Verification items for the finished model (mm, model axes). A direction names the side the tool comes from. Give positions to 0.01 mm unless a question says otherwise; leave off trailing zeros. Order: outer loops, then holes, each group sorted by start corner. A loop starts at its lowest first (then second) coordinate and runs counter-clockwise, first axis right, second up. Notation, with made-up numbers: (-9.75, -2.75) - (1.25, -2.75) arc R15 ccw to (1.25, 12.25) - close; hole circle Ø5 at (83.25, 37.25). An arc over 180 degrees is marked (long way). Answer as a JSON object with one key per item and string values. Group by question number.
(1) Section check C-C (x = 1.05). Count the separate pieces of the cut face and the enclosed holes in it, then the cut area to 3 significant figures.
(2) Access from +Z, -Z, +X, -X, +Y, -Y to the whole of each face (thin tool, end or side, straight path). Record for faces 4 (the face through (1.01, 17.4, -18.43)), 5 (the face through (1.01, 29.42, 14.59)), 6 (the face through (0.99, 45.43, 20.85)).
(3) Mould release check, pull along Z, two halves, no side actions. Record for faces 1 (the face through (1, 26, 2)), 2 (the face through (1, 15, -19)), 3 (the face through (0, 33, 0)): +Z half, -Z half, draft (parallel to the pull), parting line (faces both ways), or undercut.
(4) Depth check by flat-ended pin: pin 1 Ø1 at (x, z) = (0.5, -33) entering from +Y; pin 2 Ø0.6 at (x, y) = (1.5, 43) entering from +Z; pin 3 Ø1 at (x, z) = (1, -25.5) entering from -Y. Enter the tip coordinate at first touch or a pass-through.
(5) Thickness scan on line 1 (Z direction, x = 0.15, y = 23.5); line 2 (Z direction, x = 1.2, y = 19.5); line 3 (Y direction, x = 0.85, z = -15). Record the ranges inside material, lowest first.
(6) Section check B-B (y = 51). Record the boundary of the cut face in (x, z), then the cut area to 3 significant figures.
(7) Section check D-D (z = -3.1). Record the boundary of the cut face in (x, y), then the cut area to 3 significant figures.
(8) Section check A-A (y = 21.5). Record the boundary of the cut face in (x, z), then the cut area to 3 significant figures.
```python
from build123d import *

# Parameters (mm, degrees)
EXTRUDE_1_DEPTH        = 2
HOLE_WIZARD_M3_1_D     = 3.2
HOLE_WIZARD_M3_2_D     = 3.2
CHAMFER_1_SIZE         = 15
FILLET_1_R             = 2
CHAMFER_2_SIZE         = 10
SKETCH_6_W             = 8
SKETCH_6_H             = 39
CUT_EXTRUDE_1_DEPTH    = 100
FILLET_2_R             = 1
FILLET_3_R             = 2
FILLET_2_OF_MIRROR_2_R = 1
FILLET_3_OF_MIRROR_2_R = 2
SKETCH_8_R             = 1
CUT_EXTRUDE_2_DEPTH    = 10
FILLET_4_R             = 1
FILLET_5_R             = 10
FILLET_6_R             = 1


with BuildPart() as part:
    # 草图1 → 凸台-拉伸1 (new body)
    with BuildSketch(Plane(origin=(0, 0, 0), x_dir=(0, 0, -1), z_dir=(1, 0, 0))):
        Polygon((0, 50), (26, 50), (26, 54), (32, 54), (32, 50), (35, 50), (35, 30), (14, 30), (14, 18), (19, 18), (19, 0), (0, 0), align=None)
    extrude_1 = extrude(amount=EXTRUDE_1_DEPTH)

    # 镜向1: 凸台-拉伸1 across plane
    add(extrude_1.mirror(Plane(origin=(2, 0, 0), x_dir=(1, 0, 0), z_dir=(0, 0, -1))))

    # M3 间隙孔1 (through all)
    with Locations(Plane(origin=(2, 0, 0), x_dir=(0, 0, -1), z_dir=(1, 0, 0))):
        with Locations((-15.25, 44), (-15.25, 13.5), (15.25, 13.5), (15.25, 44)):
            Hole(HOLE_WIZARD_M3_1_D / 2)

    # M3 间隙孔2 (through all)
    with Locations(Plane(origin=(2, 0, 0), x_dir=(0, 0, -1), z_dir=(1, 0, 0))):
        with Locations((-3.1, 3), (3.1, 3)):
            Hole(HOLE_WIZARD_M3_2_D / 2)

    # 倒角1
    chamfer_1_edges = [part.edges().sort_by_distance(p)[0] for p in [
        (1, 30, -35),
        (1, 30, 35),
    ]]
    chamfer(chamfer_1_edges, length=CHAMFER_1_SIZE)

    # 圆角1
    fillet_1_edges = [part.edges().sort_by_distance(p)[0] for p in [
        (1, 30, -14),
        (1, 18, -14),
        (1, 18, -19),
        (1, 30, 14),
        (1, 18, 14),
        (1, 18, 19),
    ]]
    fillet(fillet_1_edges, radius=FILLET_1_R)

    # 倒角2
    chamfer_2_edges = [part.edges().sort_by_distance(p)[0] for p in [
        (1, 0, -19),
        (1, 0, 19),
    ]]
    chamfer(chamfer_2_edges, length=CHAMFER_2_SIZE)

    # 草图6 → 切除-拉伸1 (cut)
    with BuildSketch(Plane(origin=(2, 0, 0), x_dir=(0, 0, -1), z_dir=(1, 0, 0))):
        with Locations((-6, 26.5)):
            Rectangle(SKETCH_6_W, SKETCH_6_H)
        Polygon((-30.343145751, 46), (-18.343145751, 34), (-12.343145751, 34), (-20.25, 41.906854249), (-20.25, 46), (-24.343145751, 46), align=None)
    cut_extrude_1 = extrude(amount=-CUT_EXTRUDE_1_DEPTH, mode=Mode.SUBTRACT)

    # 圆角2
    fillet_2_edges = [part.edges().sort_by_distance(p)[0] for p in [
        (1, 46, 30.343145751),
        (1, 34, 12.343145751),
    ]]
    fillet(fillet_2_edges, radius=FILLET_2_R)

    # 圆角3
    fillet_3_edges = [part.edges().sort_by_distance(p)[0] for p in [
        (1, 7, 10),
        (1, 46, 10),
        (1, 46, 2),
        (1, 7, 2),
        (1, 46, 20.25),
        (1, 41.906854249, 20.25),
        (1, 34, 18.343145751),
    ]]
    fillet(fillet_3_edges, radius=FILLET_3_R)

    # 镜向2: 切除-拉伸1 across plane
    add(cut_extrude_1.mirror(Plane.XY), mode=Mode.SUBTRACT)

    # 圆角2 of 镜向2
    fillet_2_of_mirror_2_edges = [part.edges().sort_by_distance(p)[0] for p in [
        (1, 46, -30.343145751),
        (1, 34, -12.343145751),
    ]]
    fillet(fillet_2_of_mirror_2_edges, radius=FILLET_2_OF_MIRROR_2_R)

    # 圆角3 of 镜向2
    fillet_3_of_mirror_2_edges = [part.edges().sort_by_distance(p)[0] for p in [
        (1, 7, -10),
        (1, 46, -10),
        (1, 46, -2),
        (1, 7, -2),
        (1, 46, -20.25),
        (1, 41.906854249, -20.25),
        (1, 34, -18.343145751),
    ]]
    fillet(fillet_3_of_mirror_2_edges, radius=FILLET_3_OF_MIRROR_2_R)

    # 草图8 → 切除-拉伸2 (cut)
    with BuildSketch(Plane(origin=(2, 0, 0), x_dir=(0, 0, -1), z_dir=(1, 0, 0))):
        with Locations((-25, 50)):
            Circle(SKETCH_8_R)
        with Locations((-32, 51)):
            Circle(SKETCH_8_R)
        with Locations((32, 51)):
            Circle(SKETCH_8_R)
        with Locations((25, 50)):
            Circle(SKETCH_8_R)
    extrude(amount=-CUT_EXTRUDE_2_DEPTH, mode=Mode.SUBTRACT)

    # 圆角4
    fillet_4_edges = [part.edges().sort_by_distance(p)[0] for p in [
        (1, 50, -24),
        (1, 50, 24),
    ]]
    fillet(fillet_4_edges, radius=FILLET_4_R)

    # 圆角5
    fillet_5_edges = [part.edges().sort_by_distance(p)[0] for p in [
        (1, 30, -20),
        (1, 10, -19),
        (1, 0, -9),
        (1, 30, 20),
        (1, 10, 19),
        (1, 0, 9),
    ]]
    fillet(fillet_5_edges, radius=FILLET_5_R)

    # 圆角6
    fillet_6_edges = [part.edges().sort_by_distance(p)[0] for p in [
        (1, 45, 35),
        (1, 50, -35),
        (1, 50, 35),
        (1, 45, -35),
    ]]
    fillet(fillet_6_edges, radius=FILLET_6_R)


solid = part.part
```
Solutions:
{
 "1": {"separate pieces": "1", "enclosed holes": "10", "area": "1,310 mm2"},
 "2": {"face 4": "-Z, +X, -X", "face 5": "+Z, +X, -X", "face 6": "+X, -X"},
 "3": {"face 1": "undercut", "face 2": "-Z half", "face 3": "draft"},
 "4": {"pin 1": "stops at y = 50", "pin 2": "stops at z = 33.3", "pin 3": "stops at y = 35"},
 "5": {"line 1": "z = -14 to -10, -2 to 2, 10 to 14", "line 2": "z = -14.06 to -10, -2 to 2, 10 to 14.06", "line 3": "y = 6 to 11.92, 15.08 to 18.27, 29.73 to 34, 36.66 to 42.42, 45.58 to 50"},
 "6": {"outline": "(0, -31) - (2, -31) - (2, -26) - (0, -26) - close; (0, 26) - (2, 26) - (2, 31) - (0, 31) - close", "area": "20.0 mm2"},
 "7": {"outline": "(0, 0) - (2, 0) - (2, 1.4) - (0, 1.4) - close; (0, 4.6) - (2, 4.6) - (2, 7.21) - (0, 7.21) - close; (0, 45.79) - (2, 45.79) - (2, 50) - (0, 50) - close", "area": "16.5 mm2"},
 "8": {"outline": "(0, -14) - (2, -14) - (2, -10) - (0, -10) - close; (0, -2) - (2, -2) - (2, 2) - (0, 2) - close; (0, 10) - (2, 10) - (2, 14) - (0, 14) - close", "area": "24.0 mm2"}
}
